Autodesk Inventor part; units mm, degrees
ref_plane "YZ Plane" through (0, 0, 0) normal (1, 0, 0) x (0, 1, 0)
ref_plane "XZ Plane" through (0, 0, 0) normal (0, 1, 0) x (-1, 0, 0)
ref_plane "XY Plane" through (0, 0, 0) normal (0, 0, 1) x (1, 0, 0)
sketch "Sketch1" plane through (0, 0, 0) normal (0, 1, 0) x (-1, 0, 0)
  line L0 (0, 0) -> (63.5, 0)
  line L1 (63.5, 0) -> (63.5, -63.5)
  line L2 (63.5, -63.5) -> (0, -63.5)
  line L3 (0, -63.5) -> (0, 0)
  line L4 (0, -31.75) -> (31.75, -31.75)
  line L5 (31.75, -31.75) -> (31.75, -63.5)
  line L6 (31.75, -31.75) -> (12.7, -31.75)
  line L7 (31.75, -31.75) -> (50.8, -31.75) construction
  line L8 (12.7, -31.75) -> (12.7, -50.8)
  circle A0 centre (12.7, -50.8) radius 1.5875
  circle A1 centre (50.8, -50.8) radius 1.5875
  circle A2 centre (12.7, -12.7) radius 1.5875
  circle A3 centre (50.8, -12.7) radius 1.5875
  dimension "d0" = 63.5
  dimension "d1" = 63.5
  dimension "d2" = 19.05
  dimension "d3" = 180
  dimension "d4" = 19.05
  dimension "d5" = 3.175
  dimension "d8" = 38.1
  dimension "d11" = 38.1
extrude "Extrusion1" add sketch "Sketch1" along normal blind 3.175
sketch "Sketch2" plane through (0, 3.175, 0) normal (0, 1, 0) x (1, 0, 0)
  circle A0 centre (-12.7, 12.7) radius 1.5875
  line L0 (-12.7, 15.875) -> (-9.9504, 14.2875)
  line L1 (-9.9504, 14.2875) -> (-9.9504, 11.1125)
  line L2 (-9.9504, 11.1125) -> (-12.7, 9.525)
  line L3 (-12.7, 9.525) -> (-15.4496, 11.1125)
  line L4 (-15.4496, 11.1125) -> (-15.4496, 14.2875)
  line L5 (-15.4496, 14.2875) -> (-12.7, 15.875)
  circle A1 centre (-50.8, 12.7) radius 1.5875
  circle A2 centre (-12.7, 12.7) radius 1.5875
  circle A3 centre (-50.8, 50.8) radius 1.5875
  circle A4 centre (-12.7, 50.8) radius 1.5875
  line L6 (0, 63.5) -> (-63.5, 63.5)
  line L7 (-63.5, 63.5) -> (-63.5, 0)
  line L8 (-63.5, 0) -> (0, 0)
  line L9 (0, 0) -> (0, 63.5)
  line L10 (-50.8, 15.875) -> (-48.0504, 14.2875)
  line L11 (-48.0504, 11.1125) -> (-50.8, 9.525)
  line L12 (-50.8, 9.525) -> (-53.5496, 11.1125)
  line L13 (-53.5496, 11.1125) -> (-53.5496, 14.2875)
  line L14 (-53.5496, 14.2875) -> (-50.8, 15.875)
  line L15 (-48.0504, 14.2875) -> (-48.0504, 11.1125)
  line L16 (-12.7, 53.975) -> (-9.9504, 52.3875)
  line L17 (-9.9504, 49.2125) -> (-12.7, 47.625)
  line L18 (-12.7, 47.625) -> (-15.4496, 49.2125)
  line L19 (-15.4496, 49.2125) -> (-15.4496, 52.3875)
  line L20 (-15.4496, 52.3875) -> (-12.7, 53.975)
  line L21 (-9.9504, 52.3875) -> (-9.9504, 49.2125)
  line L22 (-50.8, 53.975) -> (-48.0504, 52.3875)
  line L23 (-48.0504, 49.2125) -> (-50.8, 47.625)
  line L24 (-50.8, 47.625) -> (-53.5496, 49.2125)
  line L25 (-53.5496, 49.2125) -> (-53.5496, 52.3875)
  line L26 (-53.5496, 52.3875) -> (-50.8, 53.975)
  line L27 (-48.0504, 52.3875) -> (-48.0504, 49.2125)
  dimension "d16" = 6.35
  dimension "d19" = 38.1
  dimension "d22" = 38.1
extrude "Extrusion2" add sketch "Sketch2" along normal blind 3.175 contours L9 L8 L7 L6
sketch "Sketch4" plane through (0, 6.35, 0) normal (0, 1, 0) x (1, 0, 0)
  line L0 (-31.75, 24.13) -> (-31.75, 0)
  line L1 (-31.75, 24.13) -> (-11.7475, 24.13)
  line L2 (-11.7475, 24.13) -> (-11.7475, 44.1325)
  circle A0 centre (-11.7475, 44.1325) radius 1.5875
  circle A1 centre (-51.7525, 44.1325) radius 1.5875
  circle A2 centre (-11.7475, 4.1275) radius 1.5875
  circle A3 centre (-51.7525, 4.1275) radius 1.5875
  circle A4 centre (-11.7475, 44.1325) radius 2.3812
  point P0 (0, 0)
  dimension "d41" = 20.0025
  dimension "d42" = 24.13
  dimension "d43" = 3.175
  dimension "d44" = 40.005
  dimension "d45" = 40.005
  dimension "d46" = 4.7625
extrude "Extrusion3" cut sketch "Sketch4" against normal up to surface (6.35 mm away) contours A0 | A1 | A2 | A3
sketch "Sketch5" plane through (0, 0, 0) normal (0, -1, 0) x (1, 0, 0)
  circle A0 centre (-51.7525, -4.1275) radius 1.5875
  circle A1 centre (-11.7475, -4.1275) radius 1.5875
  circle A2 centre (-51.7525, -44.1325) radius 1.5875
  circle A3 centre (-11.7475, -44.1325) radius 1.5875
  circle A4 centre (-51.7525, -4.1275) radius 2.3813
  circle A5 centre (-51.7525, -44.1325) radius 2.3812
  circle A6 centre (-11.7475, -44.1325) radius 2.3812
  circle A7 centre (-11.7475, -4.1275) radius 2.3812
  point P0 (0, 0)
  dimension "d51" = 4.7625
  dimension "d52" = 4.7625
  dimension "d53" = 4.7625
  dimension "d54" = 4.7625
extrude "Extrusion4" cut sketch "Sketch5" against normal blind 3.175 contours A0 | A1 | A2 | A3 | A4 | A5 | A6 | A7
sketch "Sketch6" plane through (0, 6.35, 0) normal (0, 1, 0) x (1, 0, 0)
  circle A0 centre (-51.7525, 4.1275) radius 1.5875
  circle A1 centre (-11.7475, 44.1325) radius 1.5875
  circle A2 centre (-11.7475, 4.1275) radius 1.5875
  circle A3 centre (-51.7525, 44.1325) radius 1.5875
  line L0 (-48.0504, 52.3875) -> (-48.0504, 49.2125)
  line L1 (-48.0504, 49.2125) -> (-50.8, 47.625)
  line L2 (-50.8, 47.625) -> (-53.5496, 49.2125)
  line L3 (-53.5496, 49.2125) -> (-53.5496, 52.3875)
  line L4 (-53.5496, 52.3875) -> (-50.8, 53.975)
  line L5 (-50.8, 53.975) -> (-48.0504, 52.3875)
  line L6 (-9.9504, 52.3875) -> (-9.9504, 49.2125)
  line L7 (-9.9504, 49.2125) -> (-12.7, 47.625)
  line L8 (-12.7, 47.625) -> (-15.4496, 49.2125)
  line L9 (-15.4496, 49.2125) -> (-15.4496, 52.3875)
  line L10 (-15.4496, 52.3875) -> (-12.7, 53.975)
  line L11 (-12.7, 53.975) -> (-9.9504, 52.3875)
  line L12 (-48.0504, 14.2875) -> (-48.0504, 11.1125)
  line L13 (-48.0504, 11.1125) -> (-50.8, 9.525)
  line L14 (-50.8, 9.525) -> (-53.5496, 11.1125)
  line L15 (-53.5496, 11.1125) -> (-53.5496, 14.2875)
  line L16 (-53.5496, 14.2875) -> (-50.8, 15.875)
  line L17 (-50.8, 15.875) -> (-48.0504, 14.2875)
  line L18 (-9.9504, 14.2875) -> (-9.9504, 11.1125)
  line L19 (-9.9504, 11.1125) -> (-12.7, 9.525)
  line L20 (-12.7, 9.525) -> (-15.4496, 11.1125)
  line L21 (-15.4496, 11.1125) -> (-15.4496, 14.2875)
  line L22 (-15.4496, 14.2875) -> (-12.7, 15.875)
  line L23 (-12.7, 15.875) -> (-9.9504, 14.2875)
  line L24 (0, 63.5) -> (-63.5, 63.5)
  line L25 (-63.5, 63.5) -> (-63.5, 0)
  line L26 (-63.5, 0) -> (0, 0)
  line L27 (0, 0) -> (0, 63.5)
  circle A4 centre (-31.75, 31.75) radius 19.0514
extrude "Extrusion5" cut sketch "Sketch6" against normal up to surface (6.35 mm away) contours A4
properties part number "lidarMount"
Input: part model. Units: mm. Frame: model coordinates. A direction names the side the tool comes from. Coordinates: 2 decimals unless noted, no trailing zeros. Loops run counter-clockwise (first coordinate to the right, second up) from the corner with the lowest first, then second, coordinate; pieces in that order, holes last.
Q1. Line query: line 1 along Z through (x, y) = (-49, 5.5); line 2 along X through (y, z) = (3.5, -15); line 3 along X through (y, z) = (1.75, -46). Output: solid intervals per line, ascending.
Results are:
line 1: z = -63.5 to -52.94, -48.66 to -39.84, -23.66 to -14.84, -10.56 to 0
line 2: x = -63.5 to -52.32, -49.28 to -40.83, -22.67 to -14.22, -11.18 to 0
line 3: x = -63.5 to -53.23, -50.28 to -44.39, -19.11 to -13.22, -10.27 to 0
Q2. Set-up query: faces 4 (the cylindrical face through (-49.63, 1.565, -51.873)), 5 (the flat face through (-52.194, 4.74, -53.17)), 6 (the cylindrical face through (-10.65, 1.57, -6.24)). Return all of +Z, -Z, +X, -X, +Y, -Y with unobstructed straight access to the full face (end or side cutting, diameter ignored); none if empty.
Results are:
face 4: +Y, -Y
face 5: +Y
face 6: -Y
Q3. Mould query, pull axis X, two halves, no side actions, for faces 1 (the flat face through (-31, 3, -63.5)), 2 (the cylindrical face through (-50.238, 4.785, -4.604)), 3 (the flat face through (-63.5, 3, -32)). Classes: +X half, -X half, draft (parallel to the pull), parting line (faces both ways), or undercut.
Results are:
face 1: draft
face 2: undercut
face 3: -X half
Q4. Section B-B, the plane z = -31.75. Return the cut outline in (x, y), and give its area (3 significant figures).
Results are:
outline: (-63.5, 0) - (-50.8, 0) - (-50.8, 6.35) - (-63.5, 6.35) - close; (-12.7, 0) - (0, 0) - (0, 6.35) - (-12.7, 6.35) - close
area: 161 mm2
Q5. Section A-A, the plane x = -31.75. Return the cut outline in (y, z).
Results are:
outline: (0, -63.5) - (6.35, -63.5) - (6.35, -50.8) - (0, -50.8) - close; (0, -12.7) - (6.35, -12.7) - (6.35, 0) - (0, 0) - close
Q6. Contact query for flat-ended pins moving along their axis: pin 1 (4 mm diameter, centred on x = -47.5, z = -27, fed in from -Y); pin 2 (1.6 mm diameter, centred on x = -13.5, z = -13.5, fed in from +Y) (3 decimals); pin 3 (4 mm diameter, centred on x = -11.75, z = -4.13, fed in from -Y) (3 decimals). Output: stop coordinate, or through.
Results are:
pin 1: passes through
pin 2: stops at y = 3.175
pin 3: stops at y = 3.175
